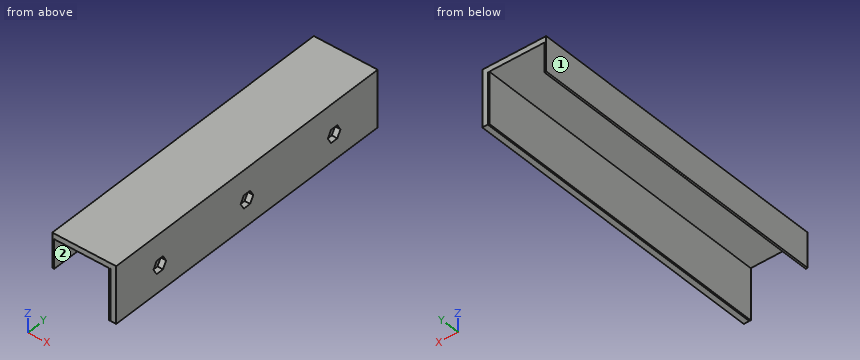
from build123d import *

# Parameters (mm, degrees)
SKETCH001_W  = 34.8
SKETCH001_H  = 170
PAD_DEPTH    = 3
SKETCH002_W  = 1
SKETCH002_H  = 170
PAD001_DEPTH = 16
SKETCH_W     = 3
SKETCH_H     = 170
SKETCH_W_2   = 0.5
PAD002_DEPTH = 28
POCKET_DEPTH = 3


with BuildPart() as part:
    # Sketch001 (on DatumPlane) → Pad (new body)
    with BuildSketch(Plane.XY.offset(28)):
        Rectangle(SKETCH001_W, SKETCH001_H)
    extrude(amount=PAD_DEPTH)

    # Sketch002 (on DatumPlane) → Pad001 (join)
    with BuildSketch(Plane.XY.offset(28)):
        with Locations((-16.9, 0)):
            Rectangle(SKETCH002_W, SKETCH002_H)
    extrude(amount=-PAD001_DEPTH)

    # Sketch (on DatumPlane) → Pad002 (join)
    with BuildSketch(Plane.XY.offset(28)):
        with Locations((15.9, 0)):
            Rectangle(SKETCH_W, SKETCH_H)
        with Locations((13.85, 0)):
            Rectangle(SKETCH_W_2, SKETCH_H)
    extrude(amount=-PAD002_DEPTH)

    # Sketch003 (on Face12 of Pad002) → Pocket (cut)
    with BuildSketch(Plane(origin=(17.4, 0, 28), x_dir=(0, 1, 0), z_dir=(1, 0, 0))):
        Polygon((-54.617073, -17.55), (-52.56748, -14), (-54.617073, -10.45), (-58.71626, -10.45), (-60.765854, -14), (-58.71626, -17.55), align=None)
        Polygon((2.049593, -17.55), (4.099187, -14), (2.049593, -10.45), (-2.049593, -10.45), (-4.099187, -14), (-2.049593, -17.55), align=None)
        Polygon((54.617073, -17.55), (58.71626, -17.55), (60.765854, -14), (58.71626, -10.45), (54.617073, -10.45), (52.56748, -14), align=None)
    extrude(amount=-POCKET_DEPTH, mode=Mode.SUBTRACT)


solid = part.part
The listing builds one solid part. Answer for the finished solid, in the listing's coordinates (mm). Face numbers are marked on the shaded views. A direction names the side the tool comes from. Round coordinates to 2 decimals unless told otherwise and drop trailing zeros. Order: outer loops, then holes, each group sorted by start corner. A loop starts at its lowest first (then second) coordinate and runs counter-clockwise, first axis right, second up. Notation, with made-up numbers: (79, 40.25) -> (136, 40.25) arc R29 ccw to (136, 73.25) -> close; hole circle Ø6 at (49.25, 53.25). An arc over 180 degrees is marked (long way). Put each result on its own line as item: value.
Q1. Which of the six approach directions +Z, -Z, +X, -X, +Y, -Y give full straight-line access (tool end or side, diameter ignored) to the marked faces 1 and 2?
Results list:
face 1: +Z, -Z, -X, +Y, -Y
face 2: -Z, +Y, -Y
Q2. Consider line 1 along X through (y, z) = (-73.5, 16); line 2 along X through (y, z) = (-47, 10); line 3 along Z through (x, y) = (1.5, -26). Determine where each line is inside the solid, lowest interval first.
Results list:
line 1: -17.4 to -16.4, 13.6 to 14.1, 14.4 to 17.4
line 2: 13.6 to 14.1, 14.4 to 17.4
line 3: 28 to 31
Q3. Section D-D, the plane z = 15.5 is taken. Write down the section's boundary in (x, y), and give its area (3 significant figures).
Results list:
outline: (-17.4, -85) -> (-16.4, -85) -> (-16.4, 85) -> (-17.4, 85) -> close; (13.6, -85) -> (14.1, -85) -> (14.1, 85) -> (13.6, 85) -> close; (14.4, -85) -> (17.4, -85) -> (17.4, -59.9) -> (14.4, -59.9) -> close; (14.4, -53.43) -> (17.4, -53.43) -> (17.4, -3.23) -> (14.4, -3.23) -> close; (14.4, 3.23) -> (17.4, 3.23) -> (17.4, 53.43) -> (14.4, 53.43) -> close; (14.4, 59.9) -> (17.4, 59.9) -> (17.4, 85) -> (14.4, 85) -> close
area: 707 mm^2
Q4. Section B-B, the plane z = 25 is taken. Write down the section's boundary in (x, y), and give its area (3 significant figures).
Results list:
outline: (-17.4, -85) -> (-16.4, -85) -> (-16.4, 85) -> (-17.4, 85) -> close; (13.6, -85) -> (14.1, -85) -> (14.1, 85) -> (13.6, 85) -> close; (14.4, -85) -> (17.4, -85) -> (17.4, 85) -> (14.4, 85) -> close
area: 765 mm^2
Q5. Section A-A, the plane z = 7.5 is taken. Write down the section's boundary in (x, y).
Results list:
outline: (13.6, -85) -> (14.1, -85) -> (14.1, 85) -> (13.6, 85) -> close; (14.4, -85) -> (17.4, -85) -> (17.4, 85) -> (14.4, 85) -> close
Q6. Each of these flat-tipped pins is pushed along its axis until it touches: P1, Ø9, axis at x = 0, y = -1.5, coming from the -Z side; P2, Ø0.5, axis at x = -17, y = 13.5, coming from the -Z side. Where does it stop, or does it pass through?
Results list:
P1: z = 28
P2: z = 12
Q7. Section C-C, the plane y = -74 is taken. Write down the section's boundary in (x, z), and give its area (3 significant figures).
Results list:
outline: (-17.4, 12) -> (-16.4, 12) -> (-16.4, 28) -> (13.6, 28) -> (13.6, 0) -> (14.1, 0) -> (14.1, 28) -> (14.4, 28) -> (14.4, 0) -> (17.4, 0) -> (17.4, 31) -> (-17.4, 31) -> close
area: 218 mm^2
